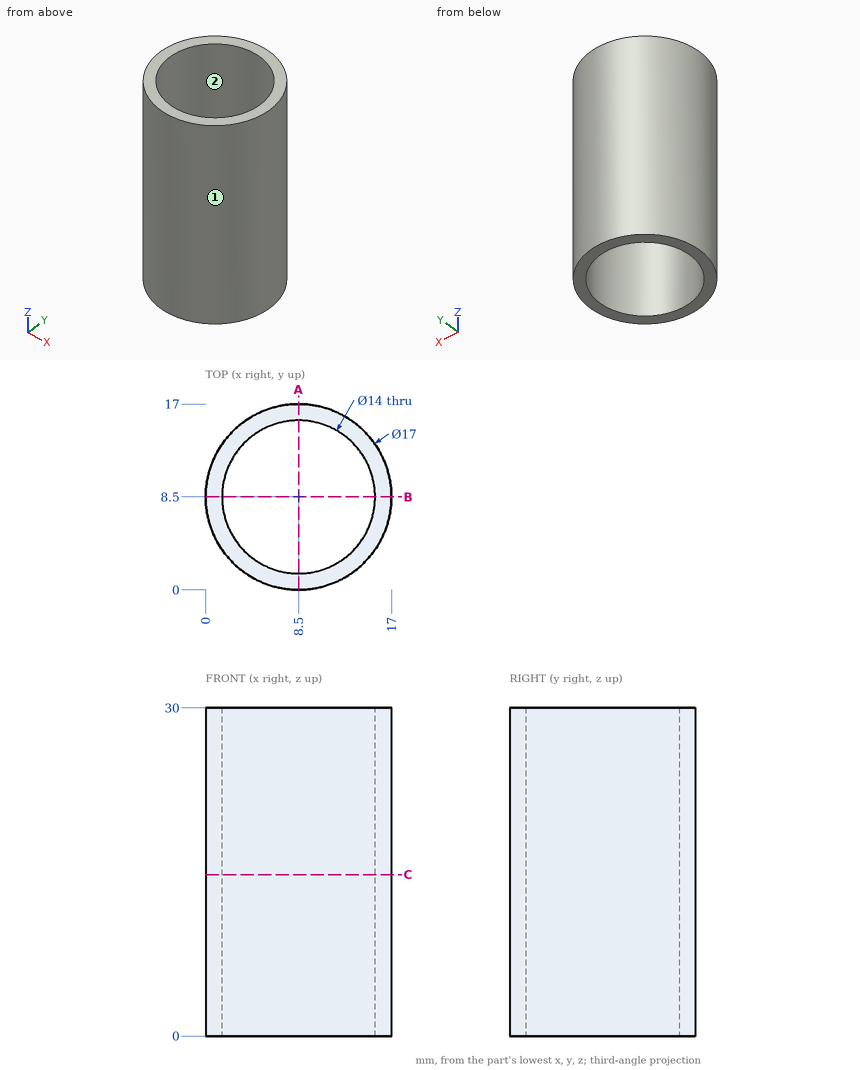
Geometry: see drawing. Coordinates: mm, zero at the bounding-box minimum. Coordinates: 2 decimals unless noted, no trailing zeros. Loops run counter-clockwise (first coordinate to the right, second up) from the corner with the lowest first, then second, coordinate; pieces in that order, holes last.
Q1. Contact query for flat-ended pins moving along their axis: pin 1 (1 mm diameter, centred on x = 12.5, z = 22, fed in from -Y); pin 2 (4 mm diameter, centred on x = 11, y = 2, fed in from +Z); pin 3 (1 mm diameter, centred on x = 9.5, z = 12.5, fed in from +Y); pin 4 (2 mm diameter, centred on x = 5.5, z = 11.5, fed in from +Y). Output: stop coordinate, or through.
Q2. Draft query along Y for the marked faces 1 and 2. Return one class per face: +Y half, -Y half, draft (parallel to the pull), parting line (faces both ways), or undercut.
Q3. Cut plane A-A (x = 8.5). Output: boundary loops of the cut face in (y, z), then the cut area to 3 significant figures.
Q4. Cut plane C-C (z = 14.75). Output: boundary loops of the cut face in (x, y).
Q5. Material intervals for line 1 (Y direction, x = 8.5, z = 6.5); line 2 (Y direction, x = 11.5, z = 18.75); line 3 (X direction, y = 2.75, z = 3.5), sorted ascending.
Working result:
1. pin 1: stops at y = 0.75
1. pin 2: stops at z = 30
1. pin 3: stops at y = 16.99
1. pin 4: stops at y = 16.76
2. face 1: parting line
2. face 2: undercut
3. outline: (0, 0) - (1.5, 0) - (1.5, 30) - (0, 30) - close; (15.5, 0) - (17, 0) - (17, 30) - (15.5, 30) - close
3. area: 90.0 mm2
4. outline: circle Ø17 at (8.5, 8.5); hole circle Ø14 at (8.5, 8.5)
5. line 1: y = 0 to 1.5, 15.5 to 17
5. line 2: y = 0.55 to 2.18, 14.82 to 16.45
5. line 3: x = 2.24 to 4.51, 12.49 to 14.76
